Input: part model. Units: mm. Frame: model coordinates. A direction names the side the tool comes from. Coordinates: 2 decimals unless noted, no trailing zeros. Loops run counter-clockwise (first coordinate to the right, second up) from the corner with the lowest first, then second, coordinate; pieces in that order, holes last. Notation, with made-up numbers: M 9,-14 L 26,-14 A31 cw 26,22 Z; hole C 66.5,30.25 d6. An arc over 180 degrees is marked long. Use a Markdown table: item, result. Add a question column.
1. Set-up query: faces 1 (the flat face through (14.75, -1, 0)), 2 (the flat face through (15.55, -1, 0)). Return all of +Z, -Z, +X, -X, +Y, -Y with unobstructed straight access to the full face (end or side cutting, diameter ignored); none if empty.
2. Line query: L1, parallel to Z at x = 1, y = -1.4; L2, parallel to X at y = -0.6, z = 0.75; L3, parallel to Y at x = -4, z = 5.5. Output: solid intervals per line, ascending. Write a range as [from, to].
3. Section A-A on y = -1.6. Output: boundary loops of the cut face in (x, z).
4. Pin query (flat end, axial travel): pin 1 (2 mm diameter, centred on x = -3.5, z = -3, fed in from -Y). Return the tip coordinate at first contact, or that it passes through.
5. Section B-B on z = 2.75. Output: boundary loops of the cut face in (x, y).
6. Draft query along Z for faces 3 (the cylindrical face through (15.009, -0.732, 11.537)), 4 (the cylindrical face through (-15.009, -0.732, -11.537)), 5 (the cylindrical face through (-14.465, -0.986, 10.949)). Return one class per face: +Z half, -Z half, draft (parallel to the pull), parting line (faces both ways), or undercut.
7. Section C-C on x = 4.5. Output: boundary loops of the cut face in (y, z), then the cut area to 4 significant figures.
```python
from build123d import *

# Parameters (mm, degrees)
SKETCH_2_W      = 29.5
SKETCH_2_H      = 22.5
LAYER_DEPTH     = 0.5
FILLET_1_R      = 1
EXTRUDE_1_DEPTH = 2.5


with BuildPart() as part:
    # 草图2 → layer (new body)
    with BuildSketch(Plane(origin=(0, 0, 0), x_dir=(1, 0, 0), z_dir=(0, 1, 0))):
        Rectangle(SKETCH_2_W, SKETCH_2_H)
    extrude(amount=LAYER_DEPTH)

    # 圆角1
    fillet_1_edges = [part.edges().sort_by_distance(p)[0] for p in [
        (14.75, 0.25, 11.25),
        (-14.75, 0.25, 11.25),
        (-14.75, 0.25, -11.25),
        (14.75, 0.25, -11.25),
    ]]
    fillet(fillet_1_edges, radius=FILLET_1_R)

    # 草图4 → 凸台-拉伸1 (add)
    with BuildSketch(Plane(origin=(0, 0.5, 0), x_dir=(1, 0, 0), z_dir=(0, 1, 0))):
        with BuildLine():
            Line((-13.75, -12.05), (13.75, -12.05))
            ThreePointArc((13.75, -12.05), (15.022792206, -11.522792206), (15.55, -10.25))
            Line((15.55, -10.25), (15.55, 10.25))
            ThreePointArc((15.55, 10.25), (15.022792206, 11.522792206), (13.75, 12.05))
            Line((13.75, 12.05), (-13.75, 12.05))
            ThreePointArc((-13.75, 12.05), (-15.022792206, 11.522792206), (-15.55, 10.25))
            Line((-15.55, 10.25), (-15.55, -10.25))
            ThreePointArc((-15.55, -10.25), (-15.022792206, -11.522792206), (-13.75, -12.05))
        make_face()
        with BuildLine():
            Line((-13.75, -11.25), (13.75, -11.25))
            ThreePointArc((13.75, -11.25), (14.457106781, -10.957106781), (14.75, -10.25))
            Line((14.75, -10.25), (14.75, 10.25))
            ThreePointArc((14.75, 10.25), (14.457106781, 10.957106781), (13.75, 11.25))
            Line((13.75, 11.25), (-13.75, 11.25))
            ThreePointArc((-13.75, 11.25), (-14.457106781, 10.957106781), (-14.75, 10.25))
            Line((-14.75, 10.25), (-14.75, -10.25))
            ThreePointArc((-14.75, -10.25), (-14.457106781, -10.957106781), (-13.75, -11.25))
        make_face(mode=Mode.SUBTRACT)
    extrude(amount=-EXTRUDE_1_DEPTH)


solid = part.part
```
Answers below:
| question | item | result |
|---|---|---|
| 1 | face 1 | -Y |
| 1 | face 2 | +Z, -Z, +X, +Y, -Y |
| 2 | L1 | z = [-12.05, -11.25], [11.25, 12.05] |
| 2 | L2 | x = [-15.55, -14.75], [14.75, 15.55] |
| 2 | L3 | y = [0, 0.5] |
| 3 | outline | M -15.55,-10.25 A1.8 ccw -13.75,-12.05 L 13.75,-12.05 A1.8 ccw 15.55,-10.25 L 15.55,10.25 A1.8 ccw 13.75,12.05 L -13.75,12.05 A1.8 ccw -15.55,10.25 Z; hole M -14.75,-10.25 A1 ccw -13.75,-11.25 L 13.75,-11.25 A1 ccw 14.75,-10.25 L 14.75,10.25 A1 ccw 13.75,11.25 L -13.75,11.25 A1 ccw -14.75,10.25 Z |
| 4 | pin 1 | stops at y = 0 |
| 5 | outline | M -15.55,-2 L -14.75,-2 L -14.75,0 L 14.75,0 L 14.75,-2 L 15.55,-2 L 15.55,0.5 L -15.55,0.5 Z |
| 6 | face 3 | +Z half |
| 6 | face 4 | -Z half |
| 6 | face 5 | undercut |
| 7 | outline | M -2,-12.05 L 0.5,-12.05 L 0.5,12.05 L -2,12.05 L -2,11.25 L 0,11.25 L 0,-11.25 L -2,-11.25 Z |
| 7 | area | 15.25 mm² |
